```python
from build123d import *

# Parameters (mm, degrees)
EXTRUDE_1_DEPTH          = 30
SKETCH_5_W               = 160
SKETCH_5_H               = 320
EXTRUDE_4_DEPTH          = 50
SKETCH_6_W               = 120
SKETCH_6_H               = 300
CUT_EXTRUDE_1_DEPTH      = 30
SKETCH_7_W               = 30
SKETCH_7_H               = 280
CUT_EXTRUDE_2_DEPTH      = 766.965155529
CUT_EXTRUDE_4_DEPTH      = 555.376568193
CUT_EXTRUDE_4_DEPTH_BACK = 555.376568193
SKETCH_10_W              = 120
SKETCH_10_H              = 180
CUT_EXTRUDE_5_DEPTH      = 766.965155601
EXTRUDE_5_DEPTH          = 80


with BuildPart() as part:
    # 草图1 → 凸台-拉伸1 (new body)
    with BuildSketch(Plane.XY):
        with BuildLine():
            Line((-550.33557047, 530.40869088), (-550.33557047, -369.59130912))
            Line((-550.33557047, -369.59130912), (-390.33557047, -369.59130912))
            Line((-390.33557047, -369.59130912), (-390.33557047, 530.40869088))
            Line((-390.33557047, 530.40869088), (-410.33557047, 530.40869088))
            Line((-410.33557047, 530.40869088), (-410.33557047, 450.40869088))
            ThreePointArc((-410.33557047, 450.40869088), (-470.33557047, 390.40869088), (-530.33557047, 450.40869088))
            Line((-530.33557047, 450.40869088), (-530.33557047, 530.40869088))
            Line((-530.33557047, 530.40869088), (-550.33557047, 530.40869088))
        make_face()
    extrude(amount=EXTRUDE_1_DEPTH)

    # 草图5 → 凸台-拉伸4 (add)
    with BuildSketch(Plane.XY.offset(30)):
        with Locations((-470.33557047, -209.59130912)):
            Rectangle(SKETCH_5_W, SKETCH_5_H)
    extrude(amount=EXTRUDE_4_DEPTH)

    # 草图6 → 切除-拉伸1 (cut)
    with BuildSketch(Plane.XY.offset(30)):
        with Locations((-470.33557047, -199.59130912)):
            Rectangle(SKETCH_6_W, SKETCH_6_H)
    extrude(amount=CUT_EXTRUDE_1_DEPTH, mode=Mode.SUBTRACT)

    # 草图7 → 切除-拉伸2 (cut, through all)
    with BuildSketch(Plane.XY.offset(30)):
        with Locations((-470.33557047, -189.59130912)):
            Rectangle(SKETCH_7_W, SKETCH_7_H)
    extrude(amount=-CUT_EXTRUDE_2_DEPTH, mode=Mode.SUBTRACT)

    # 草图9 → 切除-拉伸4 (cut, two sides: drawn at the far end of the back side and taken through both)
    with BuildSketch(Plane(origin=(-530.33557047, 0, 0), x_dir=(0, 0, -1), z_dir=(1, 0, 0)).offset(-CUT_EXTRUDE_4_DEPTH_BACK)):
        with BuildLine():
            Line((-7.5, 450.40869088), (-7.5, 520.40869088))
            ThreePointArc((-7.5, 520.40869088), (-15, 527.90869088), (-22.5, 520.40869088))
            Line((-22.5, 520.40869088), (-22.5, 450.40869088))
            ThreePointArc((-22.5, 450.40869088), (-15, 442.90869088), (-7.5, 450.40869088))
        make_face()
    extrude(amount=CUT_EXTRUDE_4_DEPTH + CUT_EXTRUDE_4_DEPTH_BACK, mode=Mode.SUBTRACT)

    # 草图10 → 切除-拉伸5 (cut, through all)
    with BuildSketch(Plane.XY.offset(30)):
        with Locations((-470.33557047, 360.40869088)):
            Rectangle(SKETCH_10_W, SKETCH_10_H)
    extrude(amount=-CUT_EXTRUDE_5_DEPTH, mode=Mode.SUBTRACT)

    # 草图11 → 凸台-拉伸5 (add)
    with BuildSketch(Plane.XY.offset(80)):
        Polygon((-550.33557047, -369.59130912), (-595.33557047, -369.59130912), (-550.33557047, -49.59130912), align=None)
        Polygon((-390.33557047, -369.59130912), (-345.33557047, -369.59130912), (-390.33557047, -49.59130912), align=None)
    extrude(amount=-EXTRUDE_5_DEPTH)


solid = part.part
```
Here's how the part is built. I have some questions about the finished solid (model axes, mm). A direction names the side the tool comes from. Round coordinates to 2 decimals unless told otherwise and drop trailing zeros. Loops run counter-clockwise (first coordinate to the right, second up) from the corner with the lowest first, then second, coordinate; pieces in that order, holes last. Notation, with made-up numbers: (-4.5, 7.5) -> (-0.5, 7.5) arc R32 ccw to (-0.5, 43.5) -> close; hole circle Ø6 at (35.5, 30.5). An arc over 180 degrees is marked (long way). Answer as CSV lines item,"result".
1. If we section it at B-B on x = -470: Please give me the cut outline in (y, z).
Final values:
outline,"(-369.59, 0) -> (-329.59, 0) -> (-329.59, 30) -> (-349.59, 30) -> (-349.59, 60) -> (-49.59, 60) -> (-49.59, 80) -> (-369.59, 80) -> close; (-49.59, 0) -> (270.41, 0) -> (270.41, 30) -> (-49.59, 30) -> close"
2. If I drill on L1, parallel to Y at x = -467.5, z = 29; L2, parallel to Z at x = -492, y = -213; L3, parallel to Z at x = -540, y = 63.5, over which ranges is the centre line in solid material (lowest first)?
Final values:
L1,"y = -369.59 to -329.59, -49.59 to 270.41"
L2,"z = 0 to 30, 60 to 80"
L3,"z = 0 to 30"
3. For pin 1 (9 mm diameter, centred on y = -202.5, z = 7.5, fed in from -X); pin 2 (9 mm diameter, centred on y = 163, z = 20.5, fed in from +X); pin 3 (15 mm diameter, centred on y = -179, z = 38, fed in from -X); pin 4 (16 mm diameter, centred on x = -397, y = 481, fed in from -Z), each with a flat end and sliding along its axis, tell me the tip position at first contact or that it passes through.
Final values:
pin 1,"stops at x = -572.47"
pin 2,"stops at x = -390.34"
pin 3,"stops at x = -569.59"
pin 4,"stops at z = 0"
4. Which directions (+Z, -Z, +X, -X, +Y, -Y) give clear straight access to the entire face, cutting with the end or side of a thin tool? Please do faces 1 (the face through (-471, -329.591, 15)), 2 (the face through (-410.336, 370, 15)), 3 (the face through (-550.336, 236, 15)).
Final values:
face 1,"-Z"
face 2,"+Z, -Z, +Y"
face 3,"+Z, -Z, -X, +Y"
5. If we section it at C-C on x = -518: Please give me the cut outline in (y, z).
Final values:
outline,"(-369.59, 0) -> (270.41, 0) -> (270.41, 30) -> (-349.59, 30) -> (-349.59, 60) -> (-49.59, 60) -> (-49.59, 80) -> (-369.59, 80) -> close"
6. If we section it at D-D on y = 25: Please give me the cut outline in (x, z).
Final values:
outline,"(-550.34, 0) -> (-390.34, 0) -> (-390.34, 30) -> (-550.34, 30) -> close"
7. If we section it at A-A on z = 15: Please give me the cut outline in (x, y).
Final values:
outline,"(-595.34, -369.59) -> (-345.34, -369.59) -> (-390.34, -49.59) -> (-390.34, 442.91) -> (-410.34, 442.91) -> (-410.34, 270.41) -> (-530.34, 270.41) -> (-530.34, 442.91) -> (-550.34, 442.91) -> (-550.34, -49.59) -> close; (-550.34, 527.91) -> (-530.34, 527.91) -> (-530.34, 530.41) -> (-550.34, 530.41) -> close; (-410.34, 527.91) -> (-390.34, 527.91) -> (-390.34, 530.41) -> (-410.34, 530.41) -> close; hole (-485.34, -329.59) -> (-455.34, -329.59) -> (-455.34, -49.59) -> (-485.34, -49.59) -> close"
8. Thinking about a two-plate mould opening in Y: for faces 4 (the face through (-530.336, -202, 45)), 5 (the face through (-540, 486, 22.5)), 6 (the face through (-540, 530.409, 15)), 7 (the face through (-455.336, -192, 15)), which applies, released by +Y, released by -Y, zero draft, split by the parting line, or undercut?
Final values:
face 4,"zero draft"
face 5,"undercut"
face 6,"released by +Y"
face 7,"undercut"
